Geometry check sheet. Reference: the model listing, model coordinates, mm. Face numbers are marked on the shaded views. A direction names the side the tool comes from. Coordinates: 2 decimals unless noted, no trailing zeros. Order: outer loops, then holes, each group sorted by start corner. A loop starts at its lowest first (then second) coordinate and runs counter-clockwise, first axis right, second up. Notation, with made-up numbers: (34.5, 48.5) - (64.5, 48.5) arc R13 ccw to (64.5, 54.5) - close; hole circle Ø11 at (39, 38.5). An arc over 180 degrees is marked (long way). One line per item, written item: value. Start each with the question number.
```python
from build123d import *

# Parameters (mm, degrees)
F1_DEPTH = 304.8
F2_W     = 762
F2_H     = 304.8
F3_DEPTH = 635


with BuildPart() as f1:
    # F0 (on Top) → F1 (new body)
    with BuildSketch(Plane.XY):
        with BuildLine():
            Line((0, -3.717796), (0, 0))
            Line((0, 0), (-1651, 0))
            Line((-1651, 0), (-1651, -1270))
            Line((-1651, -1270), (0, -1270))
            Line((0, -1270), (0, -1266.282204))
            Line((0, -1266.282204), (0, -952.5))
            ThreePointArc((0, -952.5), (-317.5, -635), (0, -317.5))
            Line((0, -317.5), (0, -3.717796))
        make_face()
        with BuildLine():
            ThreePointArc((0, -1266.282204), (631.282204, -635), (0, -3.717796))
            Line((0, -3.717796), (0, -317.5))
            ThreePointArc((0, -317.5), (224.506403, -410.493597), (317.5, -635))
            ThreePointArc((317.5, -635), (224.506403, -859.506403), (0, -952.5))
            Line((0, -952.5), (0, -1266.282204))
        make_face()
    extrude(amount=F1_DEPTH)

    # F2 (on face) → F3 (join)
    with BuildSketch(Plane.XY.offset(304.8)):
        with Locations((-1270, -152.4)):
            Rectangle(F2_W, F2_H)
    extrude(amount=F3_DEPTH)


solid = f1.part
```
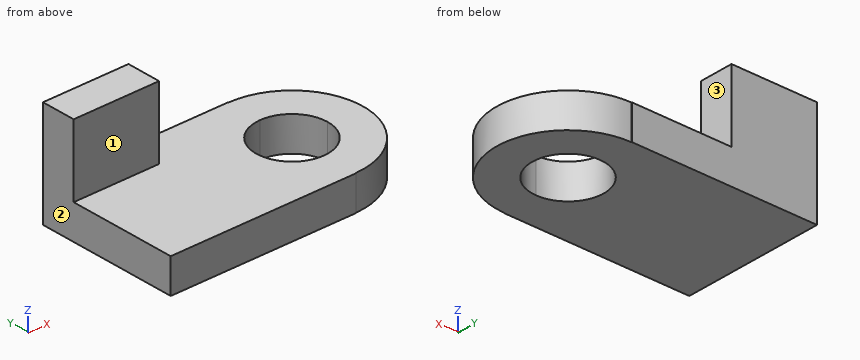
Q1. Cross-section at B-B, the plane z = 267.5. Enter the section's corners in (x, y).
Q2. Set-up check for the marked faces 1, 2 and 3: record each of +Z, -Z, +X, -X, +Y, -Y from which the full face is reachable in a straight line by a thin tool's end or side.
Q3. Material ranges on probe 1 along Z at (x, y) = (153.5, -308.5); probe 2 along X at (y, z) = (-217, 373); probe 3 along Y at (x, z) = (-1087, 529.5), recorded low to high.
Q4. Gauge pin test, flat ends, axial feed: P1, Ø10, axis at x = -1366.5, y = -1014.5, coming from the +Z side; P2, Ø1.1, axis at y = -1, z = 134.5, coming from the +X side. Record the tip position at first contact, or that the pin passes through.
Q5. Cross-section at A-A, the plane y = -837. Enter the section's corners in (x, z).
Q6. Cross-section at C-C, the plane x = -1340. Enter the section's corners in (y, z), and give its area (3 significant figures).
Q7. Cross-section at D-D, the plane y = -143. Enter the section's corners in (x, z), and give its area (3 significant figures).
Check result:
1. outline: (-1651, -1270) - (0, -1270) - (0, -1266.28) arc R631.28 ccw to (0, -3.72) - (0, 0) - (-1651, 0) - close; hole circle Ø635 at (0, -635)
2. face 1: +Z, +X, -X, -Y
2. face 2: +Z, -Z, -X, +Y, -Y
2. face 3: +Z, +X, +Y, -Y
3. probe 1: z = 0 to 304.8
3. probe 2: x = -1651 to -889
3. probe 3: y = -304.8 to 0
4. P1: stops at z = 304.8
4. P2: stops at x = 0
5. outline: (-1651, 0) - (-244.95, 0) - (-244.95, 304.8) - (-1651, 304.8) - close; (244.95, 0) - (598.09, 0) - (598.09, 304.8) - (244.95, 304.8) - close
6. outline: (-1270, 0) - (0, 0) - (0, 939.8) - (-304.8, 939.8) - (-304.8, 304.8) - (-1270, 304.8) - close
6. area: 581,000 mm2
7. outline: (-1651, 0) - (395.54, 0) - (395.54, 304.8) - (-889, 304.8) - (-889, 939.8) - (-1651, 939.8) - close
7. area: 1,110,000 mm2
